Input: dimensioned drawing with shaded views. Units: mm. Origin: part minimum x, y, z. Round coordinates to 2 decimals unless told otherwise and drop trailing zeros. Order: outer loops, then holes, each group sorted by start corner. A loop starts at its lowest first (then second) coordinate and runs counter-clockwise, first axis right, second up. Notation, with made-up numbers: M 31,8.5 L 51,8.5 A6 cw 51,12.5 Z; hole C 11,35 d3. An arc over 180 degrees is marked long. One line per question, with ' | ' between items.
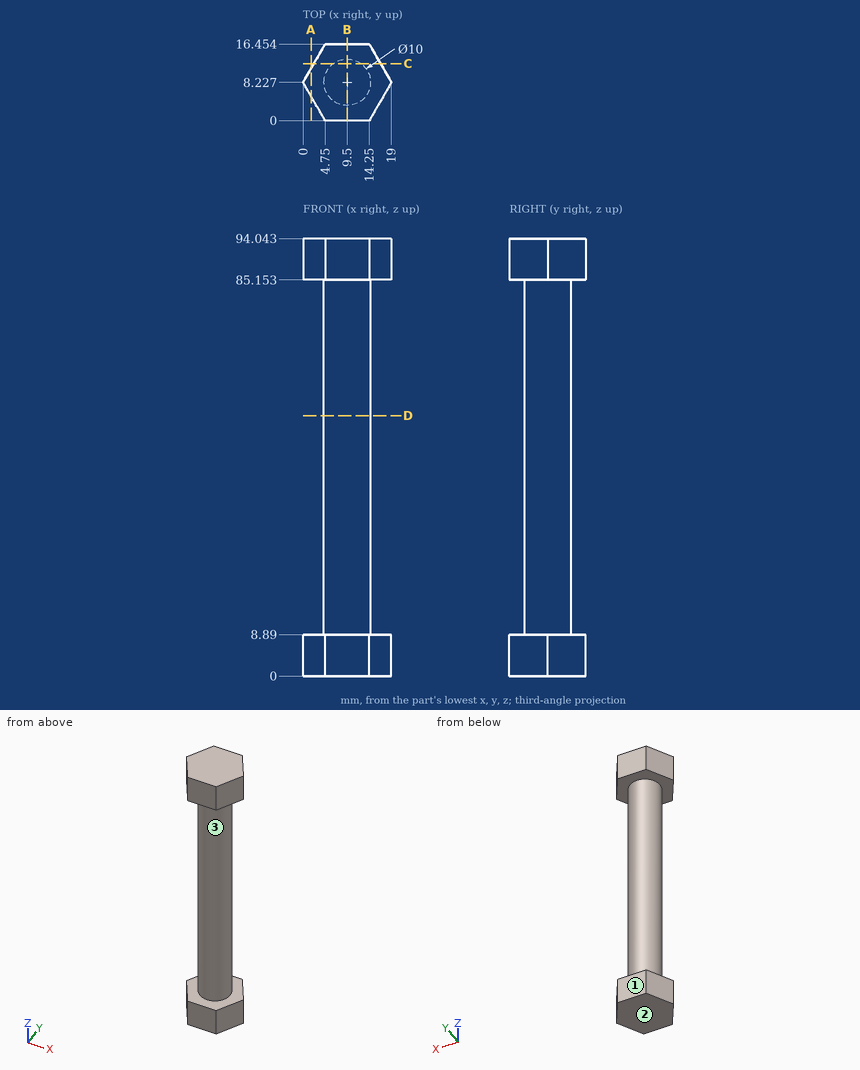
Item 1: Section query A-A, the plane x = 1.75. Return loops of the section in (y, z), plus the area to 3 significant figures.
Report:
outline: M 5.2,0 L 11.26,0 L 11.26,8.89 L 5.2,8.89 Z; M 5.2,85.15 L 11.26,85.15 L 11.26,94.04 L 5.2,94.04 Z | area: 108 mm²
Item 2: Line query: line 1 along Z through (x, y) = (16.25, 11.75); line 2 along Y through (x, z) = (9.5, 77.5); line 3 along X through (y, z) = (8.5, 33.5). Output: solid intervals per line, ascending. Write a range as from..to.
Report:
line 1: 0..8.89, 85.15..94.04 | line 2: 3.23..13.23 | line 3: 4.51..14.49
Item 3: First-contact query: pin 1 (4 mm diameter, centred on y = 9, z = 26, fed in from -X); pin 2 (4 mm diameter, centred on x = 11, y = 10, fed in from -Z); pin 3 (6 mm diameter, centred on y = 5.5, z = 81.5, fed in from +X); pin 4 (1 mm diameter, centred on x = 14.5, z = 40.5, fed in from +Y) (1 decimal). Flat tips, straight axial feed; report the tip coordinate or a pass-through.
Report:
pin 1: x = 4.5 | pin 2: z = 0 | pin 3: x = 14.5 | pin 4: y = 10.4
Item 4: Section query B-B, the plane x = 9.5. Return loops of the section in (y, z) (1 decimal).
Report:
outline: M 0,0 L 16.5,0 L 16.5,8.9 L 13.2,8.9 L 13.2,85.2 L 16.5,85.2 L 16.5,94 L 0,94 L 0,85.2 L 3.2,85.2 L 3.2,8.9 L 0,8.9 Z
Item 5: Section query C-C, the plane y = 12.25. Return loops of the section in (x, z).
Report:
outline: M 2.32,0 L 16.68,0 L 16.68,8.89 L 12.47,8.89 L 12.47,85.15 L 16.68,85.15 L 16.68,94.04 L 2.32,94.04 L 2.32,85.15 L 6.53,85.15 L 6.53,8.89 L 2.32,8.89 Z
Item 6: Section query D-D, the plane z = 56. Return loops of the section in (x, y).
Report:
outline: C 9.5,8.23 d10
Item 7: Mould query, pull axis Z, two halves, no side actions, for the marked faces 1, 2 and 3. Classes: +Z half, -Z half, draft (parallel to the pull), parting line (faces both ways), or undercut.
Report:
face 1: draft | face 2: -Z half | face 3: undercut
